```python
from build123d import *

# Parameters (mm, degrees)
SKETCH2_R           = 29.5
BOSS_EXTRUDE1_DEPTH = 7
SKETCH3_R           = 14
BOSS_EXTRUDE2_DEPTH = 3
SKETCH5_R           = 12.55
BOSS_EXTRUDE3_DEPTH = 8
SKETCH6_R           = 11
BOSS_EXTRUDE4_DEPTH = 34
SKETCH7_R           = 2.1
CUT_EXTRUDE1_DEPTH  = 33.8
SKETCH8_R           = 1.4
CUT_EXTRUDE2_DEPTH  = 19.2
SKETCH9_R           = 4.15
CUT_EXTRUDE3_DEPTH  = 9
SKETCH10_R          = 2.07
CUT_EXTRUDE4_DEPTH  = 5
SKETCH11_R          = 29.5
SKETCH11_R_2        = 26.5
BOSS_EXTRUDE5_DEPTH = 9


with BuildPart() as part:
    # Sketch2 → Boss-Extrude1 (new body)
    with BuildSketch(Plane.XY):
        Circle(SKETCH2_R)
    extrude(amount=BOSS_EXTRUDE1_DEPTH)

    # Sketch3 → Boss-Extrude2 (add)
    with BuildSketch(Plane.XY.offset(7)):
        Circle(SKETCH3_R)
    extrude(amount=BOSS_EXTRUDE2_DEPTH)

    # Sketch5 → Boss-Extrude3 (add)
    with BuildSketch(Plane.XY.offset(10)):
        Circle(SKETCH5_R)
    extrude(amount=BOSS_EXTRUDE3_DEPTH)

    # Sketch6 → Boss-Extrude4 (add)
    with BuildSketch(Plane.XY.offset(18)):
        Circle(SKETCH6_R)
    extrude(amount=BOSS_EXTRUDE4_DEPTH)

    # Sketch7 → Cut-Extrude1 (cut)
    with BuildSketch(Plane(origin=(0, 0, 0), x_dir=(-1, 0, 0), z_dir=(0, 0, -1))):
        with Locations((8, 0)):
            Circle(SKETCH7_R)
        with Locations((5.656854249, -5.656854249)):
            Circle(SKETCH7_R)
        with Locations((0, -8)):
            Circle(SKETCH7_R)
        with Locations((-5.656854249, -5.656854249)):
            Circle(SKETCH7_R)
        with Locations((-8, 0)):
            Circle(SKETCH7_R)
        with Locations((-5.656854249, 5.656854249)):
            Circle(SKETCH7_R)
        with Locations((0, 8)):
            Circle(SKETCH7_R)
        with Locations((5.656854249, 5.656854249)):
            Circle(SKETCH7_R)
    extrude(amount=-CUT_EXTRUDE1_DEPTH, mode=Mode.SUBTRACT)

    # Sketch8 → Cut-Extrude2 (cut, through all)
    with BuildSketch(Plane(origin=(0, 0, 33.8), x_dir=(-1, 0, 0), z_dir=(0, 0, -1))):
        with Locations((-8, 0)):
            Circle(SKETCH8_R)
        with Locations((-5.656854249, 5.656854249)):
            Circle(SKETCH8_R)
        with Locations((0, 8)):
            Circle(SKETCH8_R)
        with Locations((5.656854249, 5.656854249)):
            Circle(SKETCH8_R)
        with Locations((8, 0)):
            Circle(SKETCH8_R)
        with Locations((5.656854249, -5.656854249)):
            Circle(SKETCH8_R)
        with Locations((0, -8)):
            Circle(SKETCH8_R)
        with Locations((-5.656854249, -5.656854249)):
            Circle(SKETCH8_R)
    extrude(amount=-CUT_EXTRUDE2_DEPTH, mode=Mode.SUBTRACT)

    # Sketch9 → Cut-Extrude3 (cut)
    with BuildSketch(Plane.XY.offset(52)):
        Circle(SKETCH9_R)
    extrude(amount=-CUT_EXTRUDE3_DEPTH, mode=Mode.SUBTRACT)

    # Sketch10 → Cut-Extrude4 (cut)
    with BuildSketch(Plane.XY):
        with Locations((-26, 0)):
            Circle(SKETCH10_R)
        with Locations((0, 26)):
            Circle(SKETCH10_R)
        with Locations((26, 0)):
            Circle(SKETCH10_R)
        with Locations((0, -26)):
            Circle(SKETCH10_R)
    extrude(amount=CUT_EXTRUDE4_DEPTH, mode=Mode.SUBTRACT)

    # Sketch11 → Boss-Extrude5 (add)
    with BuildSketch(Plane.XY.offset(7)):
        Circle(SKETCH11_R)
        Circle(SKETCH11_R_2, mode=Mode.SUBTRACT)
    extrude(amount=BOSS_EXTRUDE5_DEPTH)


solid = part.part
```
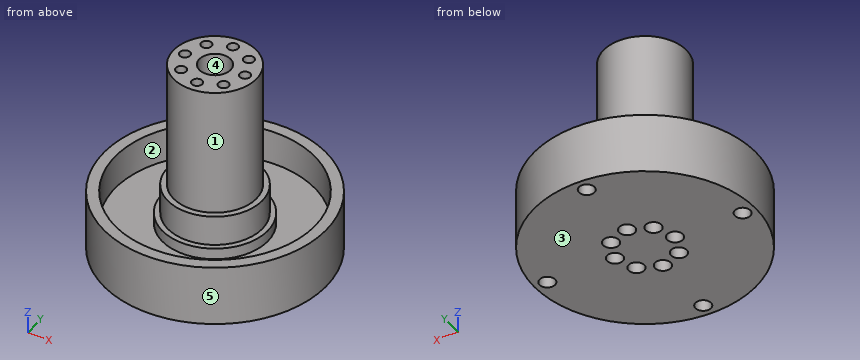
Verification items for the finished model (mm, model axes). Face numbers are marked on the shaded views. A direction names the side the tool comes from. Round coordinates to 2 decimals unless told otherwise and drop trailing zeros. Write each loop counter-clockwise with the first axis right and the second up, starting at its lowest first coordinate (ties: lowest second). Pieces come first, ordered by that corner, then holes. Notation, with made-up numbers: (46.5, 29) - (104.5, 29) arc R17 ccw to (104.5, 58) - close; hole circle Ø4 at (-39.75, 27.25). An arc over 180 degrees is marked (long way). Answer as a JSON object with one key per item and string values. Group by question number.
Q1. Go/stop test with flat-tipped pins: pin 1 Ø3.5 at (x, y) = (-8, 0) entering from -Z; pin 2 Ø1.3 at (x, y) = (5.5, -6) entering from -Z; pin 3 Ø1.5 at (x, z) = (-10.5, 13) entering from +Y; pin 4 Ø8 at (x, y) = (6.5, -0.5) entering from -Z. Record where each tip stops, or that it passes through.
Q2. Mould release check, pull along X, two halves, no side actions. Record for the marked faces 1, 2 and 3: released by +X, released by -X, zero draft, split by the parting line, or undercut.
Q3. Tool access check on the marked faces 4 and 5. Record the directions out of +Z, -Z, +X, -X, +Y, -Y that give a thin tool (end or side, any length) a straight path to the whole face; none if there is none.
Q4. Section check D-D, the plane y = 15. Enter the section's corners in (x, z).
Q5. Section check C-C, the plane x = 22.5. Enter the section's corners in (y, z).
Q6. Section check A-A, the plane y = 0. Give the number of separate pieces and of enclosed holes in the cut face, plus the area to 3 significant figures.
Q7. Thickness scan on line 1 (Y direction, x = 0, z = 9); line 2 (X direction, y = -4, z = 24); line 3 (Y direction, x = 5, z = 25). Record the ranges inside material, lowest first.
Found:
{
 "1": {"pin 1": "stops at z = 33.8", "pin 2": "passes through", "pin 3": "stops at y = 27.84", "pin 4": "stops at z = 0"},
 "2": {"face 1": "split by the parting line", "face 2": "undercut", "face 3": "zero draft"},
 "3": {"face 4": "+Z", "face 5": "+Z, -Z"},
 "4": {"outline": "(-25.4, 0) - (25.4, 0) - (25.4, 16) - (21.85, 16) - (21.85, 7) - (-21.85, 7) - (-21.85, 16) - (-25.4, 16) - close"},
 "5": {"outline": "(-19.08, 0) - (19.08, 0) - (19.08, 16) - (14, 16) - (14, 7) - (-14, 7) - (-14, 16) - (-19.08, 16) - close"},
 "6": {"separate pieces": "3", "enclosed holes": "0", "area": "998 mm^2"},
 "7": {"line 1": "y = -29.5 to -26.5, -14 to -10.1, -5.9 to 5.9, 10.1 to 14, 26.5 to 29.5", "line 2": "x = -10.25 to -6.95, -4.37 to 4.37, 6.95 to 10.25", "line 3": "y = -9.8 to -7.65, -3.66 to 3.66, 7.65 to 9.8"}
}
